Autodesk Inventor part; units mm, degrees
ref_plane "YZ Plane" through (0, 0, 0) normal (1, 0, 0) x (0, 1, 0)
ref_plane "XZ Plane" through (0, 0, 0) normal (0, 1, 0) x (-1, 0, 0)
sketch "Sketch2" plane through (0, 0, 0) normal (1, 0, 0) x (0, 1, 0)
  line L0 (0, -524.16) -> (0, 575.96)
  line L1 (0, 361.9) -> (49.78, 418.8)
  line L2 (49.78, 418.8) -> (74.08, 344.3)
  line L3 (74.08, 344.3) -> (74.08, -367)
  line L4 (74.08, -367) -> (0, -363)
  line L5 (0, -363) -> (0, 0)
  line L6 (0, 361.9) -> (0, 0)
  dimension "d0" = 361.9
  dimension "d1" = 56.9
  dimension "d2" = 49.78
  dimension "d3" = 24.3
  dimension "d4" = 74.5
  dimension "d5" = 363
  dimension "d6" = 4
  dimension "d7" = 74.08
extrude "Extrusion1" add sketch "Sketch2" along normal mid plane 154
properties part number "Enemy_hull_collision"
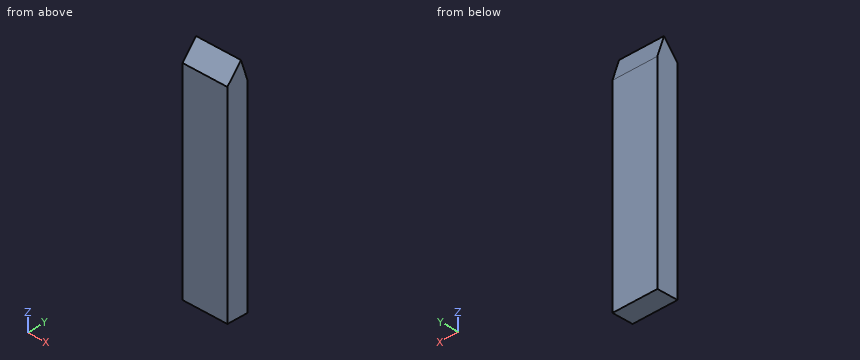
CAD build for the part. Positions are in the model's coordinates, mm. Round coordinates to 2 decimals unless told otherwise and drop trailing zeros. Write each loop counter-clockwise with the first axis right and the second up, starting at its lowest first coordinate (ties: lowest second). Pieces come first, ordered by that corner, then holes. Notation, with made-up numbers: (72, 2) - (100, 2) arc R24 ccw to (100, 14) - close; hole circle Ø1 at (45.25, 0). An arc over 180 degrees is marked (long way). Return JSON: item names as keys, results as strings. Group by question number.
Item 1: Probe probe 1 along Z at (x, y) = (-6.5, 21.5); probe 2 along Z at (x, y) = (-45, 5). List the from-to ranges inside material, lowest first.
Item 2: Band-saw the part on A-A on x = 9.5. List the corners of the cut face in (y, z).
Item 3: Flat gauge pins, fed straight in: pin 1 Ø12 at (x, z) = (21.5, -77) entering from -Y; pin 2 Ø1.5 at (x, y) = (-18.5, 19.5) entering from -Z; pin 3 Ø8 at (x, y) = (5, 58.5) entering from -Z; pin 4 Ø2 at (x, y) = (16, 48) entering from -Z. Where does each tip first touch, or does it go through?
Item 4: Band-saw the part on C-C on z = 354. List the corners of the cut face in (x, y), plus the area to 3 significant figures.
Item 5: Band-saw the part on B-B on y = 64. List the corners of the cut face in (x, z).
Resolved:
{
 "1": {"probe 1": "z = -364.16 to 386.48", "probe 2": "z = -363.27 to 367.62"},
 "2": {"outline": "(0, -363) - (74.08, -367) - (74.08, 344.3) - (49.78, 418.8) - (0, 361.9) - close"},
 "3": {"pin 1": "stops at y = 0", "pin 2": "stops at z = -364.09", "pin 3": "stops at z = -366.37", "pin 4": "stops at z = -365.65"},
 "4": {"outline": "(-77, 0) - (77, 0) - (77, 70.92) - (-77, 70.92) - close", "area": "10,900 mm²"},
 "5": {"outline": "(-77, -366.46) - (77, -366.46) - (77, 375.2) - (-77, 375.2) - close"}
}
